```python
from build123d import *

# Parameters (mm, degrees)
BASE_FLANGE1_DEPTH       = 3.175
CUT_EXTRUDE1_DEPTH       = 102.670918338
CUT_EXTRUDE2_DEPTH       = 102.670918338
F_7_0_7_DIAMETER_HOLE1_D = 7


# Sheet-metal steps are written as plain solids
with BuildPart() as part:
    # Sketch11 → Base-Flange1 (new body)
    with BuildSketch(Plane.XY.offset(3.175)):
        with BuildLine():
            Line((40.132559776, -82.017650604), (52.6, -82.017650604))
            ThreePointArc((52.6, -82.017650604), (57.832590181, -79.850240785), (60, -74.617650604))
            Line((60, -74.617650604), (60, 45))
            ThreePointArc((60, 45), (57.071067812, 52.071067812), (50, 55))
            Line((50, 55), (-50, 55))
            ThreePointArc((-50, 55), (-57.071067812, 52.071067812), (-60, 45))
            Line((-60, 45), (-60, 25))
            ThreePointArc((-60, 25), (-57.071067812, 17.928932188), (-50, 15))
            Line((-50, 15), (9.334375382, 15))
            ThreePointArc((9.334375382, 15), (15.803139956, 12.62594813), (19.200468004, 6.631016977))
            Line((19.200468004, 6.631016977), (32.831651236, -75.824603167))
            ThreePointArc((32.831651236, -75.824603167), (35.345673992, -80.260852221), (40.132559776, -82.017650604))
        make_face()
    extrude(amount=-BASE_FLANGE1_DEPTH)

    # Sketch16 → Cut-Extrude1 (cut, through all)
    with BuildSketch(Plane.XY.offset(3.175)):
        with BuildLine():
            Line((45.071829224, -20.429999447), (45.071829224, -77.229999447))
            ThreePointArc((45.071829224, -77.229999447), (46.671829224, -78.829999447), (48.271829224, -77.229999447))
            Line((48.271829224, -77.229999447), (48.271829224, -20.429999447))
            ThreePointArc((48.271829224, -20.429999447), (46.671829224, -18.829999447), (45.071829224, -20.429999447))
        make_face()
    extrude(amount=-CUT_EXTRUDE1_DEPTH, mode=Mode.SUBTRACT)

    # Sketch17 → Cut-Extrude2 (cut, through all)
    with BuildSketch(Plane(origin=(0, 0, 0), x_dir=(-1, 0, 0), z_dir=(0, 0, -1))):
        with BuildLine():
            Line((50.9, 25.770000553), (-50.9, 25.770000553))
            ThreePointArc((-50.9, 25.770000553), (-52.5, 24.170000553), (-50.9, 22.570000553))
            Line((-50.9, 22.570000553), (50.9, 22.570000553))
            ThreePointArc((50.9, 22.570000553), (52.5, 24.170000553), (50.9, 25.770000553))
        make_face()
    extrude(amount=-CUT_EXTRUDE2_DEPTH, mode=Mode.SUBTRACT)

    # Ø7.0 (7) Diameter Hole1 (through all)
    with Locations(Plane.XY.offset(3.175)):
        with Locations((35, 45), (-45, 45)):
            Hole(F_7_0_7_DIAMETER_HOLE1_D / 2)


solid = part.part
```
The model under review builds one solid part; all positions refer to its coordinate system, in mm. A direction names the side the tool comes from. Coordinates: 2 decimals unless noted, no trailing zeros. Order: outer loops, then holes, each group sorted by start corner. A loop starts at its lowest first (then second) coordinate and runs counter-clockwise, first axis right, second up. Notation, with made-up numbers: (-5, -34) -> (48, -34) arc R16 ccw to (48, -29) -> close; hole circle Ø9 at (67, -31). An arc over 180 degrees is marked (long way). Answer in a Markdown table with one row per item. Add a question column.
Item 1: We need section B-B on x = -10. Write out the cut boundary in (y, z) (3 decimals).
Item 2: We need section A-A on z = 1.1. Write out the cut boundary in (x, y).
Item 3: We need section C-C on x = 35. Write out the cut boundary in (y, z) (3 decimals), plus the area to 3 significant figures.
Item 4: Mouldability with a two-part tool opening along Y and no side actions: class faces 4 (the flat face through (60, -16, 2)), 5 (the cylindrical face through (35.29, -80.213, 1.61)), 6 (the cylindrical face through (57.15, 51.99, 1.61)), 7 (the cylindrical face through (-52.5, 24.1, 1.6)) as +Y half, -Y half, draft (parallel to the pull), parting line (faces both ways), or undercut.
Item 5: Machinability: for faces 1 (the cylindrical face through (46.64, -78.83, 1.61)), 2 (the cylindrical face through (57.77, -79.91, 1.61)), 3 (the flat face through (-21, 15, 2)), which of the approach directions +Z, -Z, +X, -X, +Y, -Y give a long, thin tool a straight path to every point of the face, cutting with its end or side? Answer none if there is none.
Item 6: We need section D-D on y = -17. Write out the cut boundary in (x, z) (3 decimals), plus the area to 3 significant figures.
Item 7: Clearance check with flat-ended pins moving along their axes: pin 1 (1.6 mm diameter, centred on x = -8, z = 1.5, fed in from -Y); pin 2 (5.5 mm diameter, centred on x = 35, y = 45, fed in from +Z); pin 3 (1 mm diameter, centred on y = -50, z = 1.5, fed in from -X); pin 4 (1 mm diameter, centred on x = 10, z = 1.5, fed in from -Y). State where each tip first meets the part, or that it passes through.
Item 8: To check wall thickness, follow probe 1 along Y at (x, z) = (-45, 1.75); probe 2 along Y at (x, z) = (-37, 1.5); probe 3 along Y at (x, z) = (34.5, 2.85). State the ranges of each line that lie inside material, in increasing order.
Final values:
| question | item | result |
|---|---|---|
| 1 | outline | (15, 0) -> (22.57, 0) -> (22.57, 3.175) -> (15, 3.175) -> close; (25.77, 0) -> (55, 0) -> (55, 3.175) -> (25.77, 3.175) -> close |
| 2 | outline | (-60, 25) arc R10 ccw to (-50, 15) -> (9.33, 15) arc R10 cw to (19.2, 6.63) -> (32.83, -75.82) arc R7.4 ccw to (40.13, -82.02) -> (52.6, -82.02) arc R7.4 ccw to (60, -74.62) -> (60, 45) arc R10 ccw to (50, 55) -> (-50, 55) arc R10 ccw to (-60, 45) -> close; hole (-50.9, 22.57) -> (50.9, 22.57) arc R1.6 ccw to (50.9, 25.77) -> (-50.9, 25.77) arc R1.6 ccw to start; hole circle Ø7 at (-45, 45); hole circle Ø7 at (35, 45); hole (45.07, -77.23) arc R1.6 ccw to (48.27, -77.23) -> (48.27, -20.43) arc R1.6 ccw to (45.07, -20.43) -> close |
| 3 | outline | (-79.948, 0) -> (22.57, 0) -> (22.57, 3.175) -> (-79.948, 3.175) -> close; (25.77, 0) -> (41.5, 0) -> (41.5, 3.175) -> (25.77, 3.175) -> close; (48.5, 0) -> (55, 0) -> (55, 3.175) -> (48.5, 3.175) -> close |
| 3 | area | 396 mm2 |
| 4 | face 4 | draft |
| 4 | face 5 | -Y half |
| 4 | face 6 | +Y half |
| 4 | face 7 | undercut |
| 5 | face 1 | +Z, -Z |
| 5 | face 2 | +Z, -Z, +X, -Y |
| 5 | face 3 | +Z, -Z, -X, -Y |
| 6 | outline | (23.107, 0) -> (60, 0) -> (60, 3.175) -> (23.107, 3.175) -> close |
| 6 | area | 117 mm2 |
| 7 | pin 1 | stops at y = 15 |
| 7 | pin 2 | passes through |
| 7 | pin 3 | stops at x = 28.48 |
| 7 | pin 4 | stops at y = 14.93 |
| 8 | probe 1 | y = 15 to 22.57, 25.77 to 41.5, 48.5 to 55 |
| 8 | probe 2 | y = 15 to 22.57, 25.77 to 55 |
| 8 | probe 3 | y = -79.42 to 22.57, 25.77 to 41.54, 48.46 to 55 |
